Read the model definition and answer for the solid it produces. Units are mm, in the model's axes. A direction names the side the tool comes from. Coordinates: 2 decimals unless noted, no trailing zeros. Order: outer loops, then holes, each group sorted by start corner. A loop starts at its lowest first (then second) coordinate and runs counter-clockwise, first axis right, second up. Notation, with made-up numbers: M 52,-6 L 70,-6 A19 ccw 70,7 Z; hole C 3.25,-27 d10. An arc over 180 degrees is marked long. Write each question's results on one line, items separated by ' | '.
```python
from build123d import *

# Parameters (mm, degrees)
BOSS_EXTRUDE1_DEPTH      = 35
BOSS_EXTRUDE1_DEPTH_BACK = 35
CUT_EXTRUDE1_DEPTH       = 13
CUT_EXTRUDE1_DEPTH_BACK  = 17
SKETCH2_W                = 20
SKETCH2_H                = 30


with BuildPart() as part:
    # Sketch1 → Boss-Extrude1 (new, two sides: drawn at the far end of the back side and taken through both)
    with BuildSketch(Plane(origin=(0, 0, 0), x_dir=(0, 0, -1), z_dir=(1, 0, 0)).offset(-BOSS_EXTRUDE1_DEPTH_BACK)):
        Polygon((0, 0), (-30.857864376, 0), (-30.857864376, 20), (-50.857864376, 20), (-50.857864376, 0), (-75.857864376, 0), (-75.857864376, 42.32233047), (-58.180194847, 60), (-10.857864376, 60), (-10.857864376, 90), (14.142135624, 90), (14.142135624, 14.142135624), align=None)
    extrude(amount=BOSS_EXTRUDE1_DEPTH + BOSS_EXTRUDE1_DEPTH_BACK)

    # Sketch2 → Cut-Extrude1 (cut, two sides: drawn at the far end of the back side and taken through both)
    with BuildSketch(Plane.XY.offset(-CUT_EXTRUDE1_DEPTH_BACK)):
        with Locations((0, 75)):
            Rectangle(SKETCH2_W, SKETCH2_H)
    extrude(amount=CUT_EXTRUDE1_DEPTH + CUT_EXTRUDE1_DEPTH_BACK, mode=Mode.SUBTRACT)


solid = part.part
```
(1) The part is cut by section C-C, the plane z = 6. Write down the section's boundary in (x, y), then the cut area to 3 significant figures.
Conclusion:
outline: M -35,0 L 35,0 L 35,90 L 10,90 L 10,60 L -10,60 L -10,90 L -35,90 Z | area: 5,700 mm²
(2) The part is cut by section B-B, the plane x = 13.5. Write down the section's boundary in (y, z), then the cut area to 3 significant figures.
Conclusion:
outline: M 0,0 L 14.14,-14.14 L 90,-14.14 L 90,10.86 L 60,10.86 L 60,58.18 L 42.32,75.86 L 0,75.86 L 0,50.86 L 20,50.86 L 20,30.86 L 0,30.86 Z | area: 5,490 mm²
(3) The part is cut by section A-A, the plane y = 7. Write down the section's boundary in (x, z).
Conclusion:
outline: M -35,-7 L 35,-7 L 35,30.86 L -35,30.86 Z; M -35,50.86 L 35,50.86 L 35,75.86 L -35,75.86 Z
(4) For faces 1 (the flat face through (0, 0, 15)), 2 (the flat face through (22, 75, 10.858)), 3 (the flat face through (0, 10, 50.858)), 4 (the flat face through (10, 75, -2)), determine the directions among +Z, -Z, +X, -X, +Y, -Y from which every point of the face is accessible in a straight line to the end or side of a thin tool.
Conclusion:
face 1: +Z, -Z, +X, -X, -Y | face 2: +Z, +X, -X, +Y | face 3: +X, -X, -Y | face 4: +Z, -Z, +Y
(5) Straight lines are drawn through the part: line 1 (Z direction, x = 21.5, y = 18.5); line 2 (Y direction, x = -13, z = 21.5); line 3 (Z direction, x = -29, y = 78). For each, find the intervals that lie inside material, in ascending order.
Conclusion:
line 1: -14.14 to 30.86, 50.86 to 75.86 | line 2: 0 to 60 | line 3: -14.14 to 10.86
(6) Given pin 1 (7.5 mm diameter, centred on x = 16.5, y = 75.5, fed in from +Z); pin 2 (1.5 mm diameter, centred on x = 16.5, z = 18.5, fed in from +Y); pin 3 (6 mm diameter, centred on x = 16.5, z = 20.5, fed in from -Y), each flat-ended and moving along its own axis, determine where each tip first touches the part or whether it passes through.
Conclusion:
pin 1: z = 10.86 | pin 2: y = 60 | pin 3: y = 0
(7) The part is cut by section D-D, the plane y = 82. Write down the section's boundary in (x, z).
Conclusion:
outline: M -35,-14.14 L -10,-14.14 L -10,10.86 L -35,10.86 Z; M 10,-14.14 L 35,-14.14 L 35,10.86 L 10,10.86 Z
